Here's the drawing with two shaded views (mm, measured from the low corner). I have some questions. A direction names the side the tool comes from. Round coordinates to 2 decimals unless told otherwise and drop trailing zeros. Loops run counter-clockwise (first coordinate to the right, second up) from the corner with the lowest first, then second, coordinate; pieces in that order, holes last.
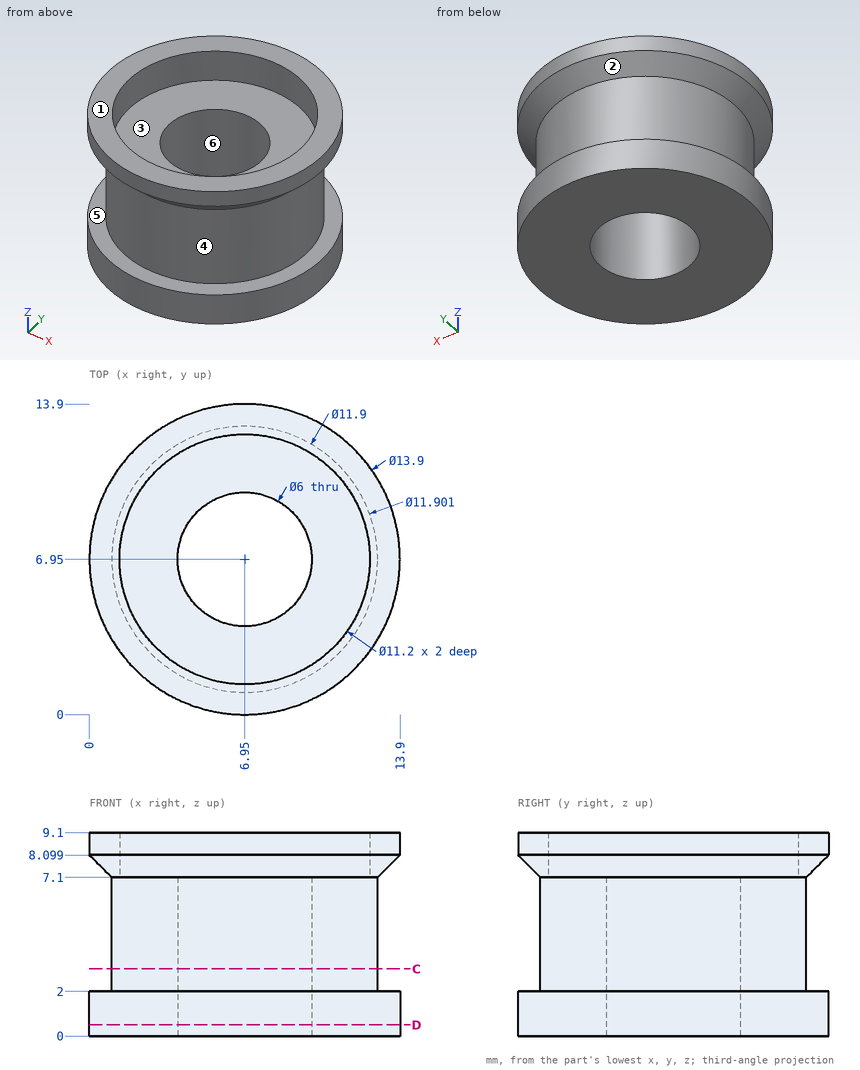
(1) If we section it at D-D, the plane z = 0.5: List the corners of the cut face in (x, y) for me.
Worked answers:
outline: circle Ø13.9 at (6.95, 6.95); hole circle Ø6 at (6.95, 6.95)
(2) Will these pins go through, and if not, where does the flat tip stop? P1, Ø1, axis at x = 9, z = 6.5, coming from the -Y side (1 decimal); P2, Ø3, axis at x = 2, z = 1.5, coming from the +Y side; P3, Ø1.5, axis at y = 8.5, z = 7, coming from the -X side (1 decimal).
Worked answers:
P1: stops at y = 1.2
P2: stops at y = 12.98
P3: stops at x = 0.5
(3) If we section it at C-C, the plane z = 3: List the corners of the cut face in (x, y) for me.
Worked answers:
outline: circle Ø11.9 at (6.95, 6.95); hole circle Ø6 at (6.95, 6.95)
(4) If I drill on line 1 (Y direction, x = 6.95, z = 8.45); line 2 (Y direction, x = 6.95, z = 4.25), over which ranges is the centre line in solid material (lowest first)?
Worked answers:
line 1: y = 0 to 1.35, 12.55 to 13.9
line 2: y = 1 to 3.95, 9.95 to 12.9
(5) For the marked faces 1, 2 and 3, which set-ups out of +Z, -Z, +X, -X, +Y, -Y let a thin tool reach every point of the face, with its end or its side?
Worked answers:
face 1: +Z, +X, -X, +Y, -Y
face 2: none
face 3: +Z
(6) If we mould it in two halves opening along Y, with no side actions, what happens to the marked faces 4, 5 and 6? For each: released by +Y, released by -Y, zero draft, split by the parting line, or undercut.
Worked answers:
face 4: split by the parting line
face 5: zero draft
face 6: undercut
